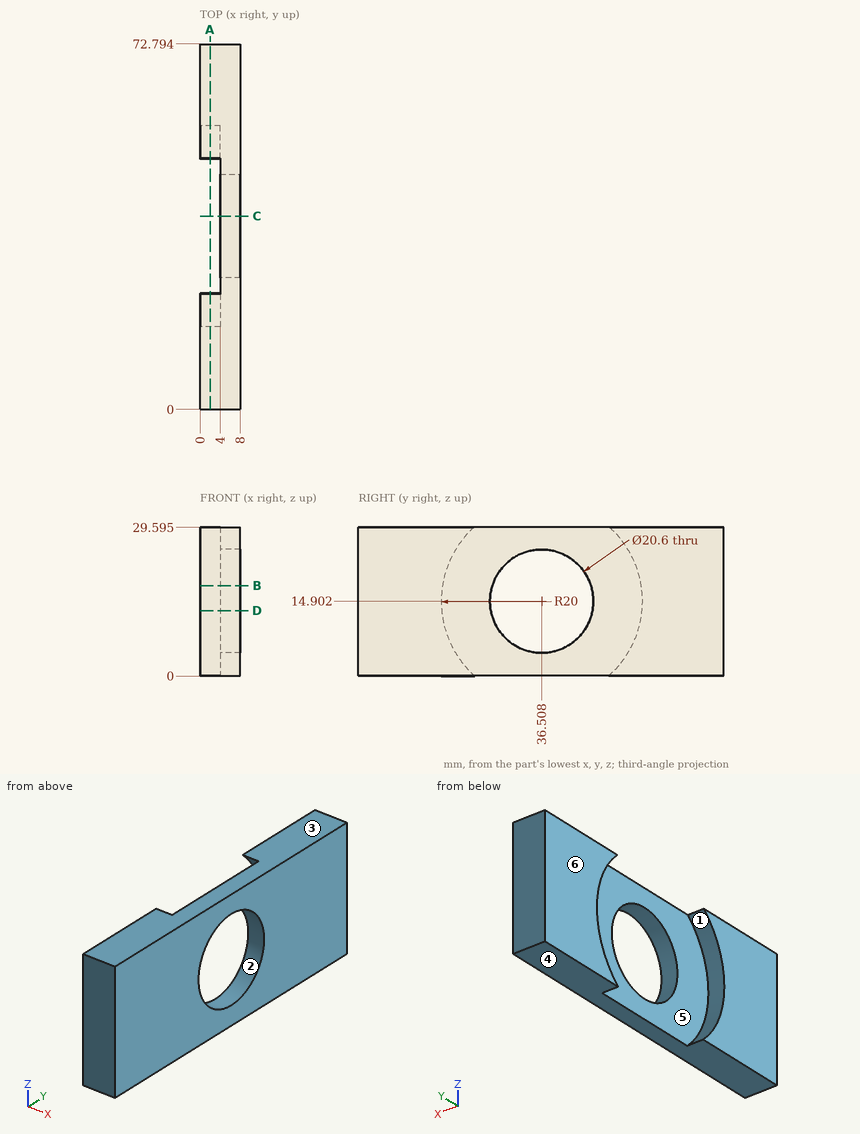
The drawing under review shows one solid part. Ordinate dimensions are in mm from its lowest x, y, z. A direction names the side the tool comes from. Coordinates: 2 decimals unless noted, no trailing zeros. Order: outer loops, then holes, each group sorted by start corner. A loop starts at its lowest first (then second) coordinate and runs counter-clockwise, first axis right, second up. Notation, with made-up numbers: M 72,14.5 L 103,14.5 A26 ccw 103,46.5 Z; hole C 24.5,87 d3. An arc over 180 degrees is marked long. Use a Markdown table: item, result.
(1) Wall thickness on probe 1 along X at (y, z) = (50.5, 24); probe 2 along Y at (x, z) = (4.5, 15.75); probe 3 along Y at (x, z) = (3.75, 13): over which ranges is each line inside the solid? List them lowest first.
Worked answers:
| item | result |
|---|---|
| probe 1 | x = 4 to 8 |
| probe 2 | y = 0 to 26.24, 46.77 to 72.79 |
| probe 3 | y = 0 to 16.6, 56.42 to 72.79 |
(2) For P1, Ø1, axis at y = 23, z = 22.5, coming from the -X side; P2, Ø12, axis at y = 55.5, z = 25, coming from the -X side, all flat-tipped, find the tip position at first contact; note any pin that passes through.
Worked answers:
| item | result |
|---|---|
| P1 | stops at x = 4 |
| P2 | stops at x = 0 |
(3) Add section A-A (x = 2). Give the boundary of the cut face in (y, z) (1 decimal), then the cut area to 3 significant figures.
Worked answers:
| item | result |
|---|---|
| outline | M 0,0 L 23.2,0 A20 cw 22.9,29.6 L 0,29.6 Z; M 49.8,0 L 72.8,0 L 72.8,29.6 L 50.1,29.6 A20 cw Z |
| area | 1,090 mm2 |
(4) Add section B-B (z = 18). Give the boundary of the cut face in (x, y) (1 decimal).
Worked answers:
| item | result |
|---|---|
| outline | M 0,0 L 8,0 L 8,26.7 L 4,26.7 L 4,16.7 L 0,16.7 Z; M 0,56.3 L 4,56.3 L 4,46.3 L 8,46.3 L 8,72.8 L 0,72.8 Z |
(5) Add section D-D (z = 13). Give the boundary of the cut face in (x, y) (1 decimal), then the cut area to 3 significant figures.
Worked answers:
| item | result |
|---|---|
| outline | M 0,0 L 8,0 L 8,26.4 L 4,26.4 L 4,16.6 L 0,16.6 Z; M 0,56.4 L 4,56.4 L 4,46.6 L 8,46.6 L 8,72.8 L 0,72.8 Z |
| area | 342 mm2 |
(6) For the marked faces 1 and 2, list the 3-axis set-ups (+Z, -Z, +X, -X, +Y, -Y) from which the entire face can be reached by the end or side of a thin tool; tool diameter is ignored.
Worked answers:
| item | result |
|---|---|
| face 1 | -X |
| face 2 | +X, -X |
(7) Draft analysis for pull direction Z (two halves, no side actions). For the marked faces 3, 4, 5 and 6, state which applies: released by +Z, released by -Z, zero draft, split by the parting line, or undercut.
Worked answers:
| item | result |
|---|---|
| face 3 | released by +Z |
| face 4 | released by -Z |
| face 5 | undercut |
| face 6 | zero draft |
(8) Add section C-C (y = 38.5). Give the boundary of the cut face in (x, z) (1 decimal).
Worked answers:
| item | result |
|---|---|
| outline | M 4,0 L 8,0 L 8,4.8 L 4,4.8 Z; M 4,25 L 8,25 L 8,29.6 L 4,29.6 Z |
